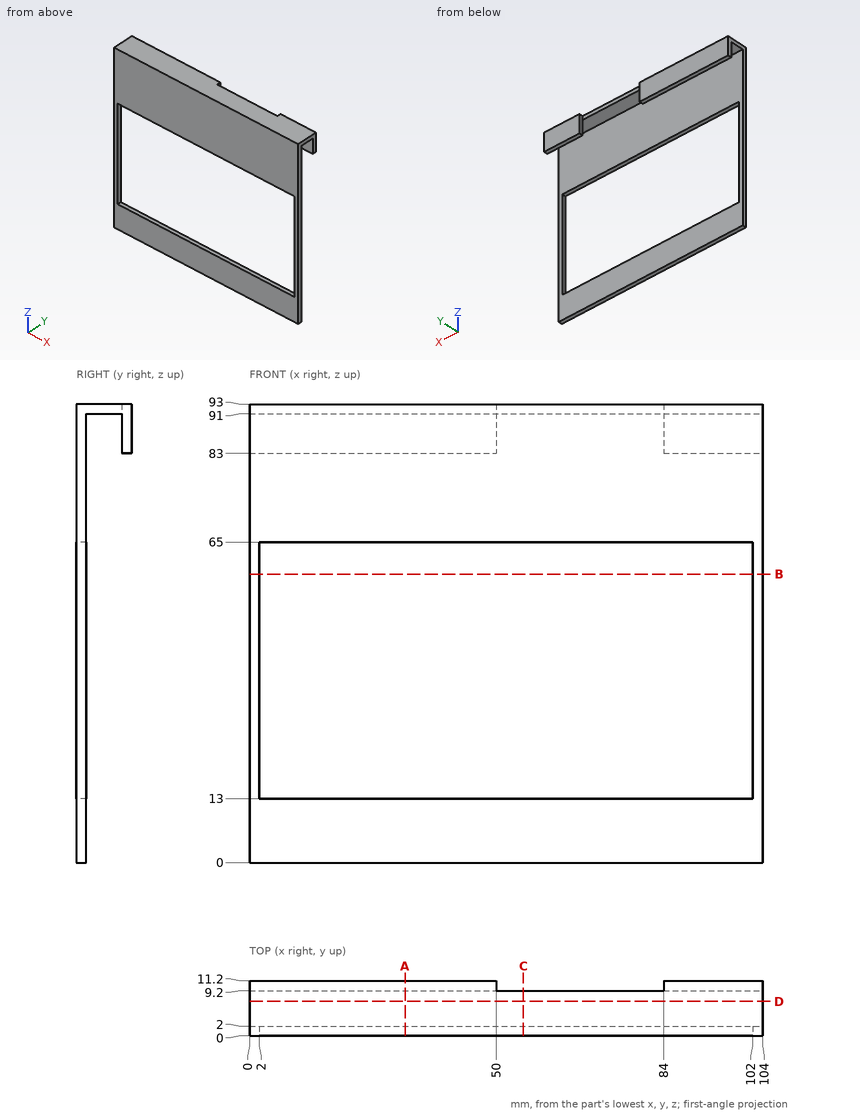
Geometry: see drawing. Coordinates: mm, zero at the bounding-box minimum. Give positions to 0.01 mm unless a question says otherwise; leave off trailing zeros. Write each loop counter-clockwise with the first axis right and the second up, starting at its lowest first coordinate (ties: lowest second). Pieces come first, ordered by that corner, then holes. Notation, with made-up numbers: M 75,33 L 88,33 A27 ccw 88,63 Z; hole C 56,-4 d2. An arc over 180 degrees is marked long. Answer as a JSON object with one key per item and string values.
Q1. Cut plane C-C, the plane x = 55.5. Return the cut outline in (y, z).
Geometry check:
{"outline": "M 0,0 L 2,0 L 2,13 L 0,13 Z; M 0,65 L 2,65 L 2,91 L 9.2,91 L 9.2,93 L 0,93 Z"}
Q2. Ray query, line 1 along Z through (x, y) = (63.5, 1.75); line 2 along X through (y, z) = (1.5, 19.5); line 3 along X through (y, z) = (10.75, 86). Return the intervals inside material, ascending.
Geometry check:
{"line 1": "z = 0 to 13, 65 to 93", "line 2": "x = 0 to 2, 102 to 104", "line 3": "x = 0 to 50, 84 to 104"}
Q3. Cut plane B-B, the plane z = 58.5. Return the cut outline in (x, y).
Geometry check:
{"outline": "M 0,0 L 2,0 L 2,2 L 0,2 Z; M 102,0 L 104,0 L 104,2 L 102,2 Z"}
Q4. Cut plane D-D, the plane y = 7. Return the cut outline in (x, z).
Geometry check:
{"outline": "M 0,91 L 104,91 L 104,93 L 0,93 Z"}
Q5. Cut plane A-A, the plane x = 31.5. Return the cut outline in (y, z), then the cut area to 3 significant figures.
Geometry check:
{"outline": "M 0,0 L 2,0 L 2,13 L 0,13 Z; M 0,65 L 2,65 L 2,91 L 9.2,91 L 9.2,83 L 11.2,83 L 11.2,93 L 0,93 Z", "area": "116 mm^2"}
Q6. Contact query for flat-ended pins moving along their axis: P1, Ø1.6, axis at y = 1.5, z = 37.5, coming from the -X side; P2, Ø1, axis at x = 72, z = 91.5, coming from the +Y side; P3, Ø1.5, axis at x = 15, z = 68, coming from the +Y side; P4, Ø4, axis at y = 4.5, z = 78.5, coming from the +X side. Output: stop coordinate, or through.
Geometry check:
{"P1": "stops at x = 0", "P2": "stops at y = 9.2", "P3": "stops at y = 2", "P4": "passes through"}
